Answer from the drawing. Dimensions are ordinates in mm from the lowest x, y and z of the part. A direction names the side the tool comes from. Coordinates: 2 decimals unless noted, no trailing zeros. Loops run counter-clockwise (first coordinate to the right, second up) from the corner with the lowest first, then second, coordinate; pieces in that order, holes last. Notation, with made-up numbers: (45, 64.5) - (94, 64.5) arc R19 cw to (94, 82.5) - close; hole circle Ø2 at (-32.5, 55.5). An arc over 180 degrees is marked (long way). Use one line per item in the form item = value. Start each with the question number.
1) A cutting plane is placed at A-A (x = 25.4). Give the vertices of the cut face in (y, z), and give its area (3 significant figures).
2) Which of the six approach directions +Z, -Z, +X, -X, +Y, -Y give full straight-line access (tool end or side, diameter ignored) to the marked faces 1 and 2?
3) Each of these flat-tipped pins is pushed along its axis until it touches: P1, Ø4, axis at y = 158, z = 3.5, coming from the -X side; P2, Ø4, axis at x = 33, z = 12.5, coming from the +Y side; P3, Ø9, axis at x = 25.4, z = 12.7, coming from the -Y side; P4, Ø2, axis at y = 57.5, z = 16, coming from the -X side. Where does it stop, or does it pass through?
4) Consider line 1 (Y direction, x = 148, z = 12.7); line 2 (Z direction, x = 151, y = 228); line 3 (Y direction, x = 134, z = 15.25). Determine where each line is inside the solid, lowest interval first.
5) A cutting plane is placed at D-D (x = 154). Give the vertices of the cut face in (y, z).
6) A cutting plane is placed at C-C (z = 12.7). Give the vertices of the cut face in (x, y), and give its area (3 significant figures).
7) A cutting plane is placed at B-B (y = 228.6). Give the vertices of the cut face in (x, z).
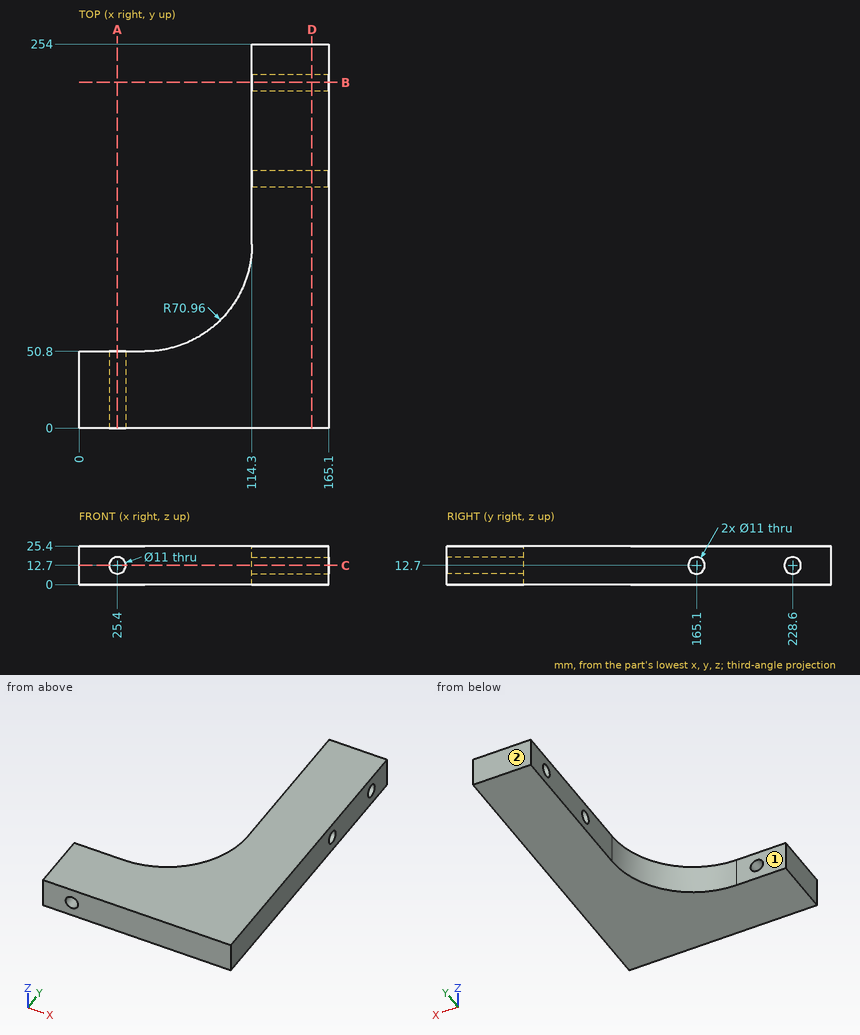
Found:
q1.outline = (0, 0) - (50.8, 0) - (50.8, 7.2) - (0, 7.2) - close; (0, 18.2) - (50.8, 18.2) - (50.8, 25.4) - (0, 25.4) - close
q1.area = 732 mm^2
q2.face_1 = +Z, -Z, -X, +Y
q2.face_2 = +Z, -Z, +X, -X, +Y
q3.P1 = 114.3
q3.P2 = 50.8
q3.P3 = through
q3.P4 = 71.2
q4.line_1 = 0 to 159.6, 170.6 to 223.1, 234.1 to 254
q4.line_2 = 0 to 7.23, 18.17 to 25.4
q4.line_3 = 0 to 160.23, 169.97 to 223.73, 233.47 to 254
q5.outline = (0, 0) - (254, 0) - (254, 25.4) - (0, 25.4) - close; hole circle Ø11 at (165.1, 12.7); hole circle Ø11 at (228.6, 12.7)
q6.outline = (0, 0) - (19.9, 0) - (19.9, 50.8) - (0, 50.8) - close; (30.9, 0) - (165.1, 0) - (165.1, 159.6) - (114.3, 159.6) - (114.3, 121.76) arc R70.96 cw to (43.34, 50.8) - (30.9, 50.8) - close; (114.3, 170.6) - (165.1, 170.6) - (165.1, 223.1) - (114.3, 223.1) - close; (114.3, 234.1) - (165.1, 234.1) - (165.1, 254) - (114.3, 254) - close
q6.area = 18,100 mm^2
q7.outline = (114.3, 0) - (165.1, 0) - (165.1, 7.2) - (114.3, 7.2) - close; (114.3, 18.2) - (165.1, 18.2) - (165.1, 25.4) - (114.3, 25.4) - close
